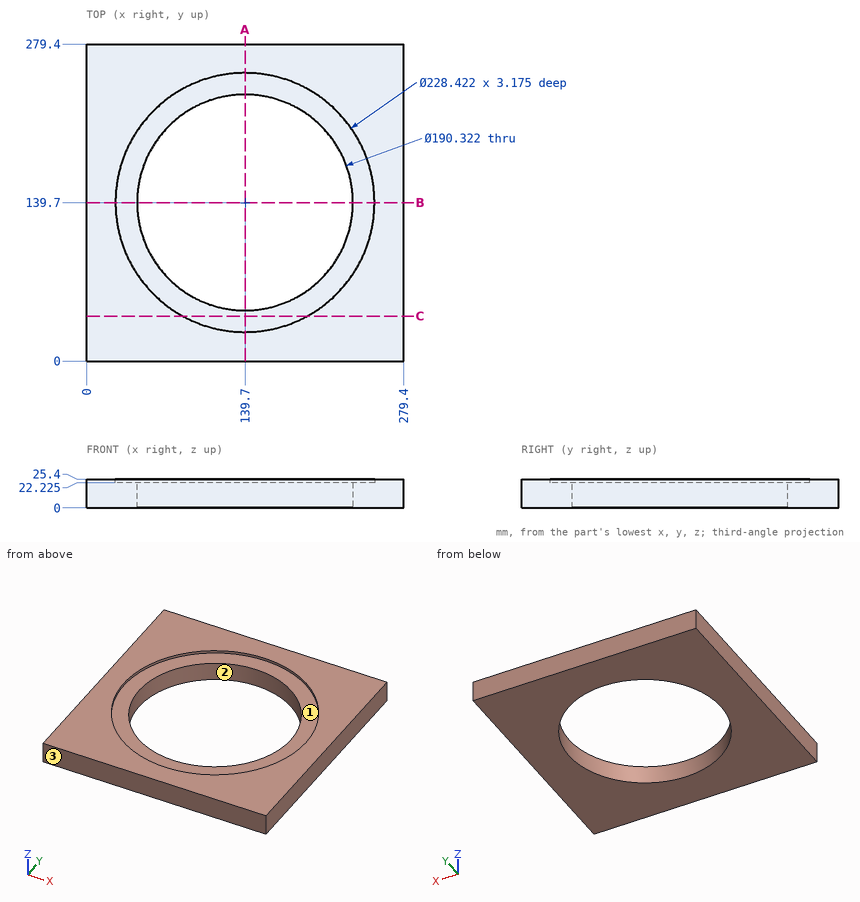
The figure shows three views and two pictorial views of one solid part (mm, origin at its lowest corner). Answer the questions. Give positions to 0.01 mm unless a question says otherwise; leave off trailing zeros. Order: outer loops, then holes, each group sorted by start corner. A loop starts at its lowest first (then second) coordinate and runs counter-clockwise, first axis right, second up. Notation, with made-up numbers: (38, 19) -> (97, 19) arc R11 cw to (97, 38) -> close; hole circle Ø1 at (6, -16). An arc over 180 degrees is marked (long way). One line per item, written item: value.
1) Determine the mould class of the marked faces 1, 2 and 3 for opening direction X: pulls with the +X half, pulls with the -X half, needs draft (parallel to the pull), parting line crosses it, or undercut.
Reported:
face 1: undercut
face 2: undercut
face 3: needs draft
2) Find the intervals of material crossed by line 1 (Y direction, x = 139.7, z = 23.6); line 2 (Y direction, x = 139.7, z = 10.75); line 3 (X direction, y = 147, z = 8.25), in increasing order.
Reported:
line 1: y = 0 to 25.49, 253.91 to 279.4
line 2: y = 0 to 44.54, 234.86 to 279.4
line 3: x = 0 to 44.82, 234.58 to 279.4
3) Find section A-A, the plane x = 139.7. Determine the outline of the cut face in (y, z) (1 decimal), plus the area to 3 significant figures.
Reported:
outline: (0, 0) -> (44.5, 0) -> (44.5, 22.2) -> (25.5, 22.2) -> (25.5, 25.4) -> (0, 25.4) -> close; (234.9, 0) -> (279.4, 0) -> (279.4, 25.4) -> (253.9, 25.4) -> (253.9, 22.2) -> (234.9, 22.2) -> close
area: 2,140 mm^2
4) Find section C-C, the plane y = 39.5. Determine the outline of the cut face in (x, z) (3 decimals), plus the area to 3 significant figures.
Reported:
outline: (0, 0) -> (279.4, 0) -> (279.4, 25.4) -> (194.51, 25.4) -> (194.51, 22.225) -> (84.89, 22.225) -> (84.89, 25.4) -> (0, 25.4) -> close
area: 6,750 mm^2
